Input: part model. Units: mm. Frame: model coordinates. A direction names the side the tool comes from. Coordinates: 2 decimals unless noted, no trailing zeros. Loops run counter-clockwise (first coordinate to the right, second up) from the corner with the lowest first, then second, coordinate; pieces in that order, holes last. Notation, with made-up numbers: (-16.5, 29) - (19.5, 29) arc R23 cw to (19.5, 52) - close; hole circle Ø1 at (82, -11.5). An arc over 180 degrees is marked (long way). Use one line per item in the form item = value.
from build123d import *

# Parameters (mm, degrees)
SKETCH27_W                 = 69.85
SKETCH27_H                 = 152.4
BOSS_EXTRUDE4_DEPTH        = 25.4
SKETCH28_W                 = 22.225
SKETCH28_H                 = 139.7
CUT_EXTRUDE5_DEPTH         = 26.4
SKETCH30_OUTSIDE_W         = 87.834
SKETCH30_OUTSIDE_H         = 189.434
CUT_EXTRUDE6_DEPTH         = 35.925
CUT_EXTRUDE6_DEPTH_BACK    = 35.925
F_3_8_CLEARANCE_HOLE4_D    = 10.31748
AUXILIARY_MOUNTING_HOLES_D = 10.31748


with BuildPart() as part:
    # Sketch27 → Boss-Extrude4 (new body, symmetric)
    with BuildSketch(Plane.XY):
        Rectangle(SKETCH27_W, SKETCH27_H)
    extrude(amount=BOSS_EXTRUDE4_DEPTH, both=True)

    # Sketch28 → Cut-Extrude5 (cut, symmetric)
    with BuildSketch(Plane.XY):
        with Locations((23.8125, 6.35)):
            Rectangle(SKETCH28_W, SKETCH28_H)
    cut_extrude5 = extrude(amount=CUT_EXTRUDE5_DEPTH, both=True, mode=Mode.SUBTRACT)

    # Mirror1: Cut-Extrude5 across plane
    add(cut_extrude5.mirror(Plane(origin=(0, 0, 0), x_dir=(0, 0, 1), z_dir=(1, 0, 0))), mode=Mode.SUBTRACT)

    # Sketch30 outside → Cut-Extrude6 (cut, two sides)
    with BuildSketch(Plane(origin=(0, 0, 0), x_dir=(0, 0, -1), z_dir=(1, 0, 0))) as cut_extrude6_sk:
        Rectangle(SKETCH30_OUTSIDE_W, SKETCH30_OUTSIDE_H)
        Polygon((-25.4, 25.4), (-25.4, -76.2), (25.4, -76.2), (25.4, 25.4), (12.7, 76.2), (-12.7, 76.2), align=None, mode=Mode.SUBTRACT)
    extrude(amount=CUT_EXTRUDE6_DEPTH, mode=Mode.SUBTRACT)
    extrude(cut_extrude6_sk.sketch, amount=-CUT_EXTRUDE6_DEPTH_BACK, mode=Mode.SUBTRACT)

    # 3/8 Clearance Hole4 (through all)
    with Locations(Plane.ZY.offset(34.925)):
        with Locations((25.4, 82.55), (0, 57.15)):
            Hole(F_3_8_CLEARANCE_HOLE4_D / 2)

    # Auxiliary Mounting Holes (through all)
    with Locations(Plane(origin=(12.7, 0, 0), x_dir=(0, 0, -1), z_dir=(1, 0, 0))):
        with Locations((-12.7, -19.05), (12.7, -19.05)):
            Hole(AUXILIARY_MOUNTING_HOLES_D / 2)


solid = part.part
Q1. Cut plane D-D, the plane z = 15. Return loops of the section in (x, y) (3 decimals).
Check values:
outline = (-34.925, -76.2) - (34.925, -76.2) - (34.925, -63.5) - (12.7, -63.5) - (12.7, -23.668) - (-12.7, -23.668) - (-12.7, -63.5) - (-34.925, -63.5) - close; (-12.7, -14.432) - (12.7, -14.432) - (12.7, 67) - (-12.7, 67) - close
Q2. Cut plane A-A, the plane z = 0. Return loops of the section in (x, y) (3 decimals), then the cut area to 3 significant figures.
Check values:
outline = (-34.925, -76.2) - (34.925, -76.2) - (34.925, -63.5) - (12.7, -63.5) - (12.7, 51.991) - (-12.7, 51.991) - (-12.7, -63.5) - (-34.925, -63.5) - close; (-12.7, 62.309) - (12.7, 62.309) - (12.7, 76.2) - (-12.7, 76.2) - close
area = 4,170 mm²
Q3. Ray query, line 1 along Y through (x, z) = (3, 0); line 2 along X through (y, z) = (24, 5); line 3 along Y through (x, z) = (21.5, 1.5). Return the intervals inside material, ascending. Write a range as [from, to].
Check values:
line_1 = [-76.2, 51.99], [62.31, 76.2]
line_2 = [-12.7, 12.7]
line_3 = [-76.2, -63.5]
Q4. Cut plane C-C, the plane x = -28.5. Return loops of the section in (y, z).
Check values:
outline = (-76.2, -25.4) - (-63.5, -25.4) - (-63.5, 25.4) - (-76.2, 25.4) - close
Q5. Set-up query: faces 1 (the flat face through (12.7, 5, 0)), 2 (the flat face through (-24, -63.5, 0)), 3 (the cylindrical face through (0.178, 52.114, 1.118)). Return all of +Z, -Z, +X, -X, +Y, -Y with unobstructed straight access to the full face (end or side cutting, diameter ignored); none if empty.
Check values:
face_1 = +Z, -Z, +X, +Y
face_2 = +Z, -Z, -X, +Y
face_3 = +X, -X
Q6. Cut plane B-B, the plane y = -19.05. Return loops of the section in (x, z).
Check values:
outline = (-12.7, -25.4) - (12.7, -25.4) - (12.7, -17.86) - (-12.7, -17.86) - close; (-12.7, -7.54) - (12.7, -7.54) - (12.7, 7.54) - (-12.7, 7.54) - close; (-12.7, 17.86) - (12.7, 17.86) - (12.7, 25.4) - (-12.7, 25.4) - close
Q7. First-contact query: P1, Ø11, axis at x = -19.5, z = -12.5, coming from the +Y side; P2, Ø1.5, axis at y = -13, z = -15, coming from the +X side; P3, Ø16.5, axis at y = 57.15, z = 0, coming from the -X side. Flat tips, straight axial feed; report the tip coordinate or a pass-through.
Check values:
P1 = -63.5
P2 = 12.7
P3 = -12.7
Q8. Pull-direction query (Y, two-part tool) for faces 4 (the flat face through (0, -36, 25.4)), 5 (the cylindrical face through (-0.18, -15.56, -16.5)), 6 (the flat face through (0, -76.2, 0)); classes: pulls with the +Y half, pulls with the -Y half, needs draft (parallel to the pull), parting line crosses it, or undercut.
Check values:
face_4 = needs draft
face_5 = undercut
face_6 = pulls with the -Y half
